The listing builds one solid part. Answer for the finished solid, in the listing's coordinates (mm). Face numbers are marked on the shaded views. A direction names the side the tool comes from. Round coordinates to 2 decimals unless told otherwise and drop trailing zeros. Write each loop counter-clockwise with the first axis right and the second up, starting at its lowest first coordinate (ties: lowest second). Pieces come first, ordered by that corner, then holes. Notation, with made-up numbers: M -15,60 L 19,60 A27 cw 19,83 Z; hole C 12.25,-24.75 d3. An arc over 180 degrees is marked long. Answer as CSV lines item,"result". Start each with the question number.
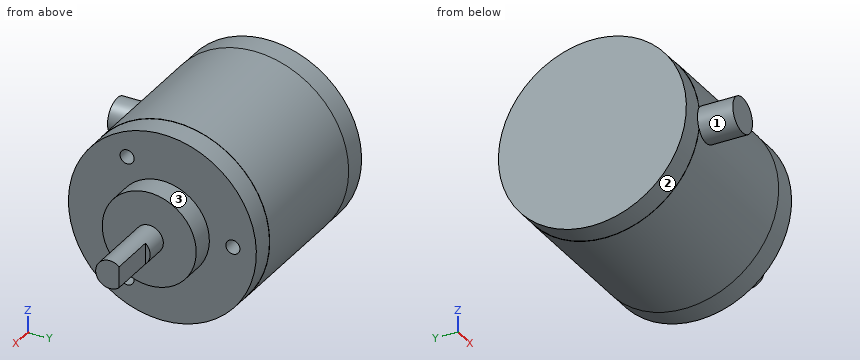
from build123d import *

# Parameters (mm, degrees)
CROQUIS1_R                  = 20
SALIENTE_EXTRUIR1_DEPTH     = 40
CROQUIS2_R                  = 10
SALIENTE_EXTRUIR2_DEPTH     = 5
CROQUIS4_R                  = 1.5
CORTAR_EXTRUIR1_DEPTH       = 5
CROQUIS5_R                  = 3
SALIENTE_EXTRUIR3_DEPTH     = 15
CORTAR_EXTRUIR2_START       = -10
CORTAR_EXTRUIR2_DEPTH       = 10
SALIENTE_EXTRUIR4_START     = -27.5
SALIENTE_EXTRUIR4_OUTLINE_R = 3.75
SALIENTE_EXTRUIR4_DEPTH     = 7.854707334
SALIENTE_EXTRUIR4_START_2   = 3
SALIENTE_EXTRUIR4_2_DEPTH   = 10
SALIENTE_EXTRUIR6_START     = 5
SALIENTE_EXTRUIR6_OUTLINE_R = 20.05
SALIENTE_EXTRUIR6_DEPTH     = 30


with BuildPart() as part:
    # Croquis1 → Saliente-Extruir1 (new body)
    with BuildSketch(Plane(origin=(0, 0, 0), x_dir=(0, 0, -1), z_dir=(1, 0, 0))):
        Circle(CROQUIS1_R)
    extrude(amount=SALIENTE_EXTRUIR1_DEPTH)

    # Croquis2 → Saliente-Extruir2 (add)
    with BuildSketch(Plane(origin=(40, 0, 0), x_dir=(0, 0, -1), z_dir=(1, 0, 0))):
        Circle(CROQUIS2_R)
    extrude(amount=SALIENTE_EXTRUIR2_DEPTH)

    # Croquis4 → Cortar-Extruir1 (cut)
    with BuildSketch(Plane(origin=(40, 0, 0), x_dir=(0, 0, -1), z_dir=(1, 0, 0))):
        with Locations((0, 15)):
            Circle(CROQUIS4_R)
        with Locations((12.990381057, -7.5)):
            Circle(CROQUIS4_R)
        with Locations((-12.990381057, -7.5)):
            Circle(CROQUIS4_R)
    extrude(amount=-CORTAR_EXTRUIR1_DEPTH, mode=Mode.SUBTRACT)

    # Croquis5 → Saliente-Extruir3 (add)
    with BuildSketch(Plane(origin=(45, 0, 0), x_dir=(0, 0, -1), z_dir=(1, 0, 0))):
        Circle(CROQUIS5_R)
    extrude(amount=SALIENTE_EXTRUIR3_DEPTH)

    # Croquis6 → Cortar-Extruir2 (cut)
    with BuildSketch(Plane(origin=(60, 0, 0), x_dir=(0, 0, -1), z_dir=(1, 0, 0)).offset(CORTAR_EXTRUIR2_START)):
        with BuildLine():
            Line((0, 2), (-2.236067977, 2))
            ThreePointArc((-2.236067977, 2), (0, 3), (2.236067977, 2))
            Line((2.236067977, 2), (0, 2))
        make_face()
    extrude(amount=CORTAR_EXTRUIR2_DEPTH, mode=Mode.SUBTRACT)



with BuildPart() as body_2:
    # Saliente-Extruir4: read off the stored shape, not the designer's step
    # Saliente-Extruir4 outline → Saliente-Extruir4 (new body)
    with BuildSketch(Plane(origin=(0, 0, 0), x_dir=(1, 0, 0), z_dir=(0, 1, 0)).offset(SALIENTE_EXTRUIR4_START)):
        with Locations((8, 0)):
            Circle(SALIENTE_EXTRUIR4_OUTLINE_R)
    extrude(amount=SALIENTE_EXTRUIR4_DEPTH)

    # Saliente-Extruir4 2 outline → Saliente-Extruir4 2 (cut)
    with BuildSketch(Plane.YZ.offset(SALIENTE_EXTRUIR4_START_2)):
        with BuildLine():
            ThreePointArc((-19.645292078, 3.749999888), (-20, 0), (-19.645292078, -3.749999888))
            Line((-19.645292078, -3.749999888), (-19.645292078, 3.749999888))
        make_face()
    extrude(amount=SALIENTE_EXTRUIR4_2_DEPTH, mode=Mode.SUBTRACT)


with BuildPart() as part_1:
    add(part.part)

    add(body_2.part)  # Saliente-Extruir6 merges body 2
    # Saliente-Extruir6: read off the stored shape, not the designer's step
    # Saliente-Extruir6 outline → Saliente-Extruir6 (add)
    with BuildSketch(Plane.YZ.offset(SALIENTE_EXTRUIR6_START)):
        Circle(SALIENTE_EXTRUIR6_OUTLINE_R)
        with BuildLine():
            ThreePointArc((-19.645240114, 3.750272106), (20, -7.213e-06), (-19.645242819, -3.750257935))
            ThreePointArc((-19.645242819, -3.750257935), (-20, 7.213e-06), (-19.645240114, 3.750272106))
        make_face(mode=Mode.SUBTRACT)
    extrude(amount=SALIENTE_EXTRUIR6_DEPTH)


solid = part_1.part
Q1. Find section B-B (y = 0). Determine the outline of the cut face in (x, z).
Q2. For the marked faces 1, 2 and 3, determine the directions among +Z, -Z, +X, -X, +Y, -Y from which every point of the face is accessible in a straight line to the end or side of a thin tool.
Q3. Straight lines are drawn through the part: L1, parallel to Z at x = 37, y = -7 (3 decimals); L2, parallel to Y at x = 37.6, z = 0; L3, parallel to Y at x = 18.5, z = 1.5. For each, find the intervals that lie inside material, in ascending order.
Q4. Each of these flat-tipped pins is pushed along its axis until it touches: P1, Ø0.9, axis at y = 15.5, z = -0.5, coming from the +X side; P2, Ø2.5, axis at y = -7, z = 13, coming from the +X side; P3, Ø12, axis at x = 33.5, z = -13.5, coming from the -Y side; P4, Ø10, axis at y = 9.5, z = -8.5, coming from the -X side. Where does it stop, or does it pass through?
Q5. Find section C-C (x = 34). Determine the outline of the cut face in (y, z).
Q6. Find section A-A (z = 0). Determine the outline of the cut face in (x, y), plus the area to 3 significant figures.
Q7. Find section D-D (x = 8). Determine the outline of the cut face in (y, z).
Reported:
1,outline,"M 0,-20 L 5,-20 L 5,-20.05 L 35,-20.05 L 35,-20 L 40,-20 L 40,-10 L 45,-10 L 45,-3 L 60,-3 L 60,3 L 45,3 L 45,10 L 40,10 L 40,20 L 35,20 L 35,20.05 L 5,20.05 L 5,20 L 0,20 Z"
2,face 1,"-Y"
2,face 2,"-X"
2,face 3,"+X"
3,L1,"z = -18.735 to -14.405, -11.576 to 11.576, 14.405 to 18.735"
3,L2,"y = -20 to 13.5, 16.5 to 20"
3,L3,"y = -19.99 to 19.99"
4,P1,"stops at x = 35"
4,P2,"stops at x = 40"
4,P3,"stops at y = -18.59"
4,P4,"stops at x = 0"
5,outline,"C 0,0 d40.1"
6,outline,"M 0,-20 L 4.25,-20 L 4.25,-27.5 L 11.75,-27.5 L 11.75,-20.05 L 35,-20.05 L 35,-20 L 40,-20 L 40,-10 L 45,-10 L 45,-3 L 60,-3 L 60,2 L 50,2 L 50,3 L 45,3 L 45,10 L 40,10 L 40,13.5 L 35,13.5 L 35,16.5 L 40,16.5 L 40,20 L 35,20 L 35,20.05 L 5,20.05 L 5,20 L 0,20 Z"
6,area,"1,820 mm2"
7,outline,"M -27.5,-3.75 L -19.7,-3.75 A20.05 ccw long -19.7,3.75 L -27.5,3.75 Z"
